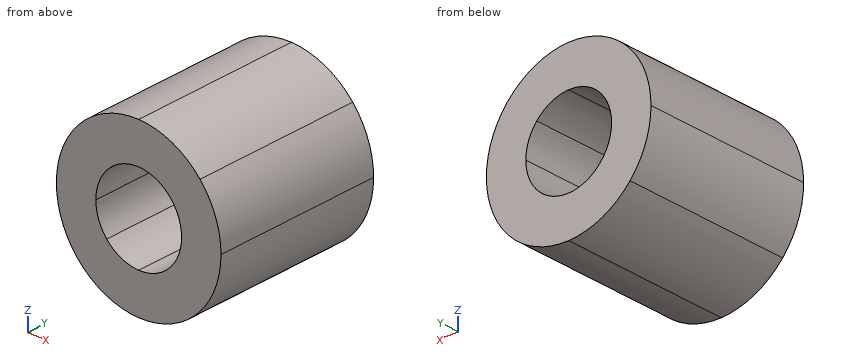
from build123d import *

# Parameters (mm, degrees)
F1_DEPTH = 25


with BuildPart() as f1:
    # F0 (on Front) → F1 (new body)
    with BuildSketch(Plane.XZ):
        with BuildLine():
            ThreePointArc((-4.3394231509, 4.8722430533), (-2.3216701125, 6.0974743576), (0, 6.5245188062))
            Line((0, 6.5245188062), (0, 12.5245188062))
            ThreePointArc((0, 12.5245188062), (-4.4566966316, 11.7047608459), (-8.3299916017, 9.3527969743))
            Line((-8.3299916017, 9.3527969743), (-4.3394231509, 4.8722430533))
        make_face()
        with BuildLine():
            Line((-12.5245188062, 0), (-6.5245188062, 0))
            ThreePointArc((-6.5245188062, 0), (-5.9532341466, 2.6698967861), (-4.3394231509, 4.8722430533))
            Line((-4.3394231509, 4.8722430533), (-8.3299916017, 9.3527969743))
            ThreePointArc((-8.3299916017, 9.3527969743), (-11.4278761762, 5.1251553564), (-12.5245188062, 0))
        make_face()
        with BuildLine():
            ThreePointArc((-4.8633482309, -4.3493895707), (-6.0950944474, -2.3279109368), (-6.5245188062, 0))
            Line((-6.5245188062, 0), (-12.5245188062, 0))
            ThreePointArc((-12.5245188062, 0), (-11.7001923513, -4.468676568), (-9.3357224016, -8.3491232214))
            Line((-9.3357224016, -8.3491232214), (-4.8633482309, -4.3493895707))
        make_face()
        with BuildLine():
            Line((0, -12.5245188062), (0, -6.5245188062))
            ThreePointArc((0, -6.5245188062), (-2.6638010064, -5.9559642251), (-4.8633482309, -4.3493895707))
            Line((-4.8633482309, -4.3493895707), (-9.3357224016, -8.3491232214))
            ThreePointArc((-9.3357224016, -8.3491232214), (-5.1134538487, -11.4331168569), (0, -12.5245188062))
        make_face()
        with BuildLine():
            Line((8.3299916017, -9.3527969743), (4.3394231509, -4.8722430533))
            ThreePointArc((4.3394231509, -4.8722430533), (2.3216701125, -6.0974743576), (0, -6.5245188062))
            Line((0, -6.5245188062), (0, -12.5245188062))
            ThreePointArc((0, -12.5245188062), (4.4566966316, -11.7047608459), (8.3299916017, -9.3527969743))
        make_face()
        with BuildLine():
            ThreePointArc((4.8633482309, 4.3493895707), (6.0950944474, 2.3279109368), (6.5245188062, 0))
            Line((6.5245188062, 0), (12.5245188062, 0))
            ThreePointArc((12.5245188062, 0), (11.7001923513, 4.468676568), (9.3357224016, 8.3491232214))
            Line((9.3357224016, 8.3491232214), (4.8633482309, 4.3493895707))
        make_face()
        with BuildLine():
            ThreePointArc((0, 6.5245188062), (2.6638010064, 5.9559642251), (4.8633482309, 4.3493895707))
            Line((4.8633482309, 4.3493895707), (9.3357224016, 8.3491232214))
            ThreePointArc((9.3357224016, 8.3491232214), (5.1134538487, 11.4331168569), (0, 12.5245188062))
            Line((0, 12.5245188062), (0, 6.5245188062))
        make_face()
        with BuildLine():
            Line((12.5245188062, 0), (6.5245188062, 0))
            ThreePointArc((6.5245188062, 0), (5.9532341466, -2.6698967861), (4.3394231509, -4.8722430533))
            Line((4.3394231509, -4.8722430533), (8.3299916017, -9.3527969743))
            ThreePointArc((8.3299916017, -9.3527969743), (11.4278761762, -5.1251553564), (12.5245188062, 0))
        make_face()
    extrude(amount=F1_DEPTH)


solid = f1.part
Input: part model. Units: mm. Frame: model coordinates. Round coordinates to 2 decimals unless told otherwise and drop trailing zeros. Order: outer loops, then holes, each group sorted by start corner. A loop starts at its lowest first (then second) coordinate and runs counter-clockwise, first axis right, second up. Notation, with made-up numbers: (64, 70) - (108, 70) arc R19 ccw to (108, 104) - close; hole circle Ø6 at (16.25, 39). An arc over 180 degrees is marked (long way). Answer as a JSON object with one key per item and string values. Group by question number.
(1) Cut plane C-C (x = -2.25). Return loops of the section in (y, z), then the cut area to 3 significant figures.
(2) Cut plane D-D (x = 10.5). Return loops of the section in (y, z).
(3) Cut plane A-A (y = -12.25). Return loops of the section in (x, z).
(4) Material intervals for probe 1 along Z at (x, y) = (-0.25, -17.25); probe 2 along X at (y, z) = (-10.75, -1); probe 3 along Z at (x, y) = (5.25, -11), sorted ascending. Write a range as from..to.
(5) Pin query (flat end, axial travel): P1, Ø10, axis at x = 8.5, y = -12.5, coming from the +Z side; P2, Ø3, axis at x = -2.5, y = -6, coming from the -Z side; P3, Ø6, axis at x = 9.5, y = -11.5, coming from the +Z side. Return the tip coordinate at first contact, or that it passes through.
(6) Cut plane B-B (z = -3). Return loops of the section in (x, y), then the cut area to 3 significant figures.
Here are the results:
{
 "1": {"outline": "(-25, -12.32) - (0, -12.32) - (0, -6.12) - (-25, -6.12) - close; (-25, 6.12) - (0, 6.12) - (0, 12.32) - (-25, 12.32) - close", "area": "310 mm^2"},
 "2": {"outline": "(-25, -6.83) - (0, -6.83) - (0, 6.83) - (-25, 6.83) - close"},
 "3": {"outline": "circle Ø25.05 at (0, 0); hole circle Ø13.05 at (0, 0)"},
 "4": {"probe 1": "z = -12.52..-6.52, 6.52..12.52", "probe 2": "x = -12.48..-6.45, 6.45..12.48", "probe 3": "z = -11.37..-3.87, 3.87..11.37"},
 "5": {"P1": "stops at z = 12.03", "P2": "stops at z = -12.48", "P3": "stops at z = 10.71"},
 "6": {"outline": "(-12.16, -25) - (-5.79, -25) - (-5.79, 0) - (-12.16, 0) - close; (5.79, -25) - (12.16, -25) - (12.16, 0) - (5.79, 0) - close", "area": "318 mm^2"}
}
